CAD build for the part. Positions are in the model's coordinates, mm. Face numbers are marked on the shaded views. A direction names the side the tool comes from. Round coordinates to 2 decimals unless told otherwise and drop trailing zeros. Write each loop counter-clockwise with the first axis right and the second up, starting at its lowest first coordinate (ties: lowest second). Pieces come first, ordered by that corner, then holes. Notation, with made-up numbers: (82, -18) - (110, -18) arc R31 cw to (110, 20) - close; hole circle Ø8 at (-33.5, -25.75). An arc over 180 degrees is marked (long way). Put each result on its own line as item: value. Start each with the question number.
Item 1: Cut at D-D (y = -14.5). Give the cut face in (x, z), and give its area (3 significant figures).
Item 2: Cut at C-C (x = 16.5). Give the cut face in (y, z), and give its area (3 significant figures).
Item 3: Pin check, flat tips, straight feed: pin 1 Ø8.5 at (y, z) = (-14.5, 11.5) entering from -X; pin 2 Ø1.9 at (x, y) = (29.5, 2) entering from +Z; pin 3 Ø5.5 at (x, z) = (-4.5, 12) entering from -Y; pin 4 Ø3 at (x, y) = (6, 10.5) entering from -Z. Stop position of each tip, or through.
Item 4: 3-axis set-ups, long thin cutter, end or side, ignore diameter. For the marked faces 1, 2, 3 and 4: which of +Z, -Z, +X, -X, +Y, -Y reach the whole face in a straight line?
Item 5: Cut at A-A (y = -7). Give the cut face in (x, z).
Item 6: Mould opens along X. For the marked faces 5, 6 and 7 say: released by +X, released by -X, zero draft, split by the parting line, or undercut.
Item 7: Drill centre lines: line 1 (X direction, y = -11, z = 18.5); line 2 (Z direction, x = -26, y = 7.5); line 3 (X direction, y = 8, z = 16.5). Where is each one in solid material? Low to high. Write a range as from..to.
Item 8: Cut at B-B (z = 10.5). Give the cut face in (x, y), and give its area (3 significant figures).
```python
from build123d import *

# Parameters (mm, degrees)
F0_W        = 63.5
F0_H        = 38.1
F1_DEPTH    = 6.35
F2_T1_DEPTH = 38.1
F3_W        = 50.8
F3_H        = 38.1
F4_DEPTH    = 19.05
F5_W        = 38.1
F5_H        = 7.6055689663
F6_DEPTH    = 19.05
F7_R        = 12.7
F8_DEPTH    = 25.4


# Not quite as in the source:
# - a fillet or chamfer that OpenCascade refuses, or shapes differently, is made with other operations: its cross-section is extruded or revolved along the edge and cut away or added


with BuildPart() as f1:
    # F0 (on Top) → F1 (new body)
    with BuildSketch(Plane.XY):
        Rectangle(F0_W, F0_H)
    extrude(amount=F1_DEPTH)

    # F2: fillet of radius 6.35 on 2 edges, made by hand

    # F2_s2 → F2_t1 (cut)
    with BuildSketch(Plane.XY.offset(-15.875)):
        with BuildLine():
            add(Edge.make_bspline(
                [(-25.4, 19.05), (-31.75, 19.05), (-31.75, 12.7)],
                knots=[0, 0, 0, 1, 1, 1], degree=2, weights=[1, 1, 1]))
            Line((-31.75, 12.7), (-31.75, 19.05))
            Line((-31.75, 19.05), (-25.4, 19.05))
        make_face()
        with BuildLine():
            add(Edge.make_bspline(
                [(31.75, 12.7), (31.75, 19.05), (25.4, 19.05)],
                knots=[0, 0, 0, 1, 1, 1], degree=2, weights=[1, 1, 1]))
            Line((25.4, 19.05), (31.75, 19.05))
            Line((31.75, 19.05), (31.75, 12.7))
        make_face()
    extrude(amount=F2_T1_DEPTH, mode=Mode.SUBTRACT)

    # F3 (on face) → F4 (join)
    with BuildSketch(Plane.XY.offset(6.35)):
        Rectangle(F3_W, F3_H)
    extrude(amount=F4_DEPTH)

    # F5 (on face) → F6 (cut)
    with BuildSketch(Plane.XY.offset(25.4)):
        with Locations((0, -15.2472155169)):
            Rectangle(F5_W, F5_H)
    extrude(amount=-F6_DEPTH, mode=Mode.SUBTRACT)

    # F7 (on face) → F8 (cut)
    with BuildSketch(Plane.XY.offset(25.4)):
        with Locations((0, 19.05)):
            Circle(F7_R)
    extrude(amount=-F8_DEPTH, mode=Mode.SUBTRACT)


solid = f1.part
```
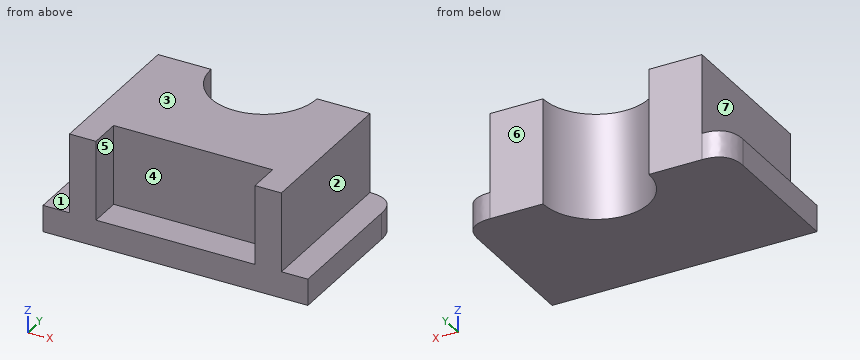
Output values:
1. outline: (-31.75, 0) - (31.75, 0) - (31.75, 6.35) - (25.4, 6.35) - (25.4, 25.4) - (19.05, 25.4) - (19.05, 6.35) - (-19.05, 6.35) - (-19.05, 25.4) - (-25.4, 25.4) - (-25.4, 6.35) - (-31.75, 6.35) - close
1. area: 645 mm2
2. outline: (-19.05, 0) - (19.05, 0) - (19.05, 25.4) - (-11.44, 25.4) - (-11.44, 6.35) - (-19.05, 6.35) - close
2. area: 823 mm2
3. pin 1: x = -25.4
3. pin 2: z = 6.35
3. pin 3: y = -11.44
3. pin 4: through
4. face 1: +Z, -X, +Y, -Y
4. face 2: +Z, +X, +Y, -Y
4. face 3: +Z, +X, -X, +Y, -Y
4. face 4: +Z, -Y
5. outline: (-31.75, 0) - (31.75, 0) - (31.75, 6.35) - (25.4, 6.35) - (25.4, 25.4) - (-25.4, 25.4) - (-25.4, 6.35) - (-31.75, 6.35) - close
6. face 5: undercut
6. face 6: zero draft
6. face 7: released by -X
7. line 1: -25.4..25.4
7. line 2: 0..6.35
7. line 3: -25.4..-6.26, 6.26..25.4
8. outline: (-25.4, -19.05) - (-19.05, -19.05) - (-19.05, -11.44) - (19.05, -11.44) - (19.05, -19.05) - (25.4, -19.05) - (25.4, 19.05) - (12.7, 19.05) arc R12.7 cw to (-12.7, 19.05) - (-25.4, 19.05) - close
8. area: 1,390 mm2
